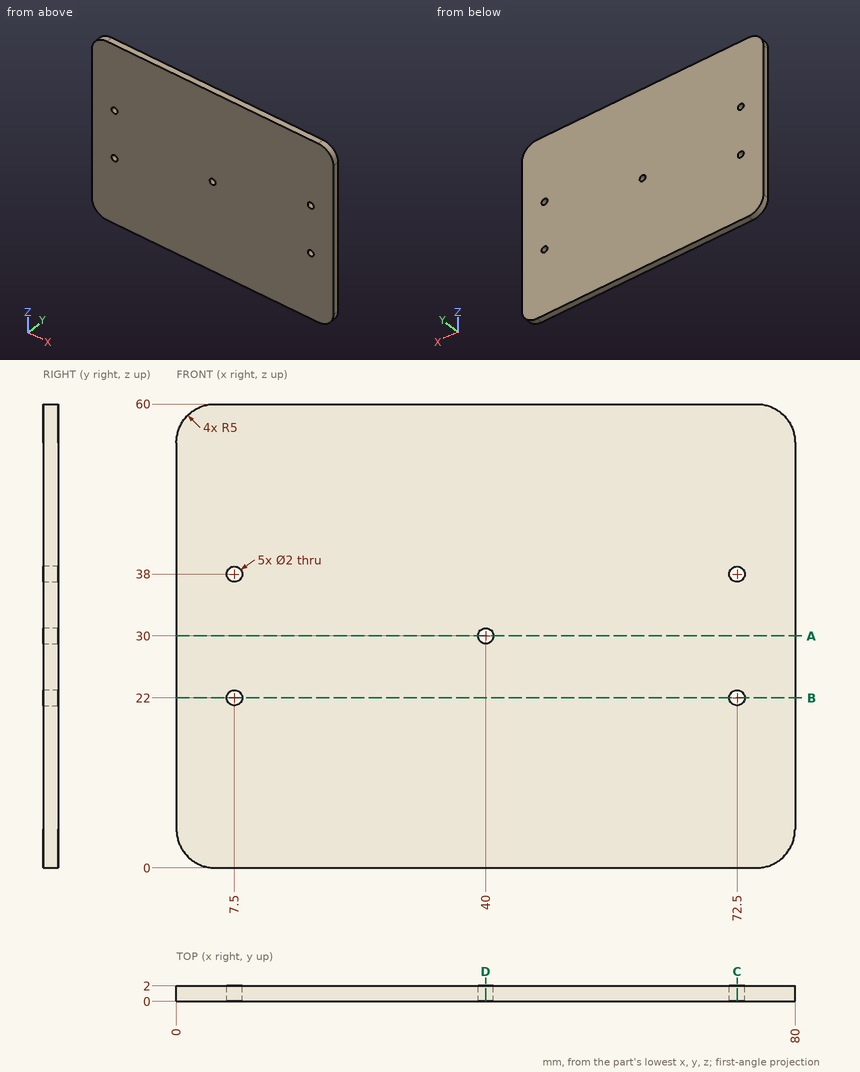
Study the drawing (mm; zero at the part's minimum x, y, z) and answer. Coordinates: 2 decimals unless noted, no trailing zeros. Order: outer loops, then holes, each group sorted by start corner. A loop starts at its lowest first (then second) coordinate and runs counter-clockwise, first axis right, second up. Notation, with made-up numbers: M 77.5,-3.5 L 105.5,-3.5 A8 cw 105.5,11.5 Z; hole C -35,64 d1. An arc over 180 degrees is marked long. Answer as a JSON object with one key per item and string values. Group by question number.
1. Straight lines are drawn through the part: line 1 (Z direction, x = 72.5, y = 0.4); line 2 (X direction, y = 0.8, z = 30); line 3 (X direction, y = 0.65, z = 38). For each, find the intervals that lie inside material, in ascending order.
2. Section D-D on x = 40 is taken. Write down the section's boundary in (y, z).
3. Section A-A on z = 30 is taken. Write down the section's boundary in (x, y).
4. Section B-B on z = 22 is taken. Write down the section's boundary in (x, y).
5. A flat-ended cylindrical pin translates along its axis: P1, Ø12, axis at x = 17.5, z = 13.5, coming from the -Y side. Find the tip coordinate at first contact, or state that the pin passes through.
6. Section C-C on x = 72.5 is taken. Write down the section's boundary in (y, z), then the cut area to 3 significant figures.
Values follow:
{
 "1": {"line 1": "0 to 21, 23 to 37, 39 to 60", "line 2": "0 to 39, 41 to 80", "line 3": "0 to 6.5, 8.5 to 71.5, 73.5 to 80"},
 "2": {"outline": "M 0,0 L 2,0 L 2,29 L 0,29 Z; M 0,31 L 2,31 L 2,60 L 0,60 Z"},
 "3": {"outline": "M 0,0 L 39,0 L 39,2 L 0,2 Z; M 41,0 L 80,0 L 80,2 L 41,2 Z"},
 "4": {"outline": "M 0,0 L 6.5,0 L 6.5,2 L 0,2 Z; M 8.5,0 L 71.5,0 L 71.5,2 L 8.5,2 Z; M 73.5,0 L 80,0 L 80,2 L 73.5,2 Z"},
 "5": {"P1": "y = 0"},
 "6": {"outline": "M 0,0 L 2,0 L 2,21 L 0,21 Z; M 0,23 L 2,23 L 2,37 L 0,37 Z; M 0,39 L 2,39 L 2,60 L 0,60 Z", "area": "112 mm2"}
}
